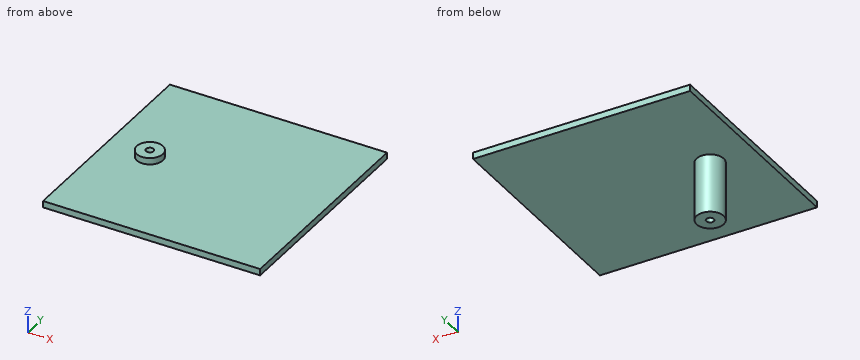
from build123d import *
from OCP.BRepFilletAPI import BRepFilletAPI_MakeChamfer

# Parameters (mm, degrees)
SKETCH1_W           = 100
SKETCH1_H           = 100
BOSS_EXTRUDE1_DEPTH = 3
SKETCH2_R           = 6.25
BOSS_EXTRUDE2_DEPTH = 30
SKETCH3_R           = 0.75
CUT_EXTRUDE1_DEPTH  = 145.568322948
SKETCH4_R           = 6
SKETCH4_R_2         = 0.75
BOSS_EXTRUDE3_DEPTH = 3
CHAMFER1_SIZE       = 1
CHAMFER1_SIZE_2     = 3


with BuildPart() as part:
    # Sketch1 → Boss-Extrude1 (new body)
    with BuildSketch(Plane.XY):
        with Locations((50, 50)):
            Rectangle(SKETCH1_W, SKETCH1_H)
    extrude(amount=BOSS_EXTRUDE1_DEPTH)

    # Sketch2 → Boss-Extrude2 (add)
    with BuildSketch(Plane.XY.offset(3)):
        with Locations((20, 50)):
            Circle(SKETCH2_R)
    extrude(amount=-BOSS_EXTRUDE2_DEPTH)

    # Sketch3 → Cut-Extrude1 (cut, through all)
    with BuildSketch(Plane(origin=(0, 0, -27), x_dir=(-1, 0, 0), z_dir=(0, 0, -1))):
        with Locations((-20, 50)):
            Circle(SKETCH3_R)
    extrude(amount=-CUT_EXTRUDE1_DEPTH, mode=Mode.SUBTRACT)

    # Sketch4 → Boss-Extrude3 (add)
    with BuildSketch(Plane.XY.offset(3)):
        with Locations(Location((20, 50, 0), (0, 0, 180))):
            Circle(SKETCH4_R)
        with Locations(Location((20, 50, 0), (0, 0, 180))):
            Circle(SKETCH4_R_2, mode=Mode.SUBTRACT)
    extrude(amount=BOSS_EXTRUDE3_DEPTH)

    # Chamfer1
    chamfer1_edges_1 = [part.edges().sort_by_distance(p)[0] for p in [
        (20.75, 50, -27),
    ]]
    chamfer1_side_1 = [part.faces().sort_by_distance(p)[0] for p in [
        (20.77, 50, -27),
    ]]
    chamfer1_edges_2 = [part.edges().sort_by_distance(p)[0] for p in [
        (20.75, 50, 6),
    ]]
    chamfer1_side_2 = [part.faces().sort_by_distance(p)[0] for p in [
        (20.77, 50, 6),
    ]]
    chamfer1 = BRepFilletAPI_MakeChamfer(part.part.solid().wrapped)
    for e in chamfer1_edges_1:
        chamfer1.Add(CHAMFER1_SIZE - 0.0001, CHAMFER1_SIZE_2 - 0.0001, e.wrapped, chamfer1_side_1[0].wrapped)
    for e in chamfer1_edges_2:
        chamfer1.Add(CHAMFER1_SIZE - 0.0001, CHAMFER1_SIZE_2 - 0.0001, e.wrapped, chamfer1_side_2[0].wrapped)
    add(Compound.cast(chamfer1.Shape()), mode=Mode.REPLACE)  # a hair under: the kernel refuses the full size


solid = part.part
Geometry: final body of the model. Coordinates: model frame, mm. Give positions to 0.01 mm unless a question says otherwise; leave off trailing zeros. Write each loop counter-clockwise with the first axis right and the second up, starting at its lowest first coordinate (ties: lowest second). Pieces come first, ordered by that corner, then holes. Notation, with made-up numbers: (42, -39.75) -> (89, -39.75) arc R25 ccw to (89, -23.75) -> close; hole circle Ø11 at (46, 24). An arc over 180 degrees is marked (long way). Answer as a JSON object with one key per item and string values.
1. Cut plane A-A on y = 46. Output: boundary loops of the cut face in (x, z).
Ans:
{"outline": "(0, 0) -> (15.2, 0) -> (15.2, -27) -> (24.8, -27) -> (24.8, 0) -> (100, 0) -> (100, 3) -> (24.47, 3) -> (24.47, 6) -> (15.53, 6) -> (15.53, 3) -> (0, 3) -> close"}
2. Contact query for flat-ended pins moving along their axis: pin 1 (1 mm diameter, centred on x = 32, y = 20, fed in from +Z); pin 2 (1 mm diameter, centred on x = 81, z = -1.5, fed in from -Y); pin 3 (5 mm diameter, centred on x = 87, y = 74, fed in from -Z); pin 4 (8 mm diameter, centred on y = 41.5, z = -18, fed in from +X). Output: stop coordinate, or through.
Ans:
{"pin 1": "stops at z = 3", "pin 2": "passes through", "pin 3": "stops at z = 0", "pin 4": "stops at x = 24.34"}
3. Cut plane C-C on z = -6. Output: boundary loops of the cut face in (x, y).
Ans:
{"outline": "circle Ø12.5 at (20, 50); hole circle Ø1.5 at (20, 50)"}
4. Cut plane B-B on x = 68.5. Output: boundary loops of the cut face in (y, z).
Ans:
{"outline": "(0, 0) -> (100, 0) -> (100, 3) -> (0, 3) -> close"}
5. Ray query, probe 1 along Y at (x, z) = (20, -18); probe 2 along X at (y, z) = (50.5, -13.5); probe 3 along Z at (x, y) = (24, 57.5). Return the intervals inside material, ascending. Write a range as from..to.
Ans:
{"probe 1": "y = 43.75..49.25, 50.75..56.25", "probe 2": "x = 13.77..19.44, 20.56..26.23", "probe 3": "z = 0..3"}
6. Cut plane D-D on x = 15.5. Output: boundary loops of the cut face in (y, z).
Ans:
{"outline": "(0, 0) -> (45.66, 0) -> (45.66, -27) -> (54.34, -27) -> (54.34, 0) -> (100, 0) -> (100, 3) -> (53.97, 3) -> (53.97, 6) -> (46.03, 6) -> (46.03, 3) -> (0, 3) -> close"}
